```python
from build123d import *

# Parameters (mm, degrees)
SKETCH010_W     = 19.05
SKETCH010_H     = 25.4
PAD006_DEPTH    = 25.4
POCKET002_DEPTH = 25.401
SKETCH012_W     = 15.05
SKETCH012_H     = 23.4
POCKET003_DEPTH = 23.4
POCKET004_DEPTH = 19.051
FILLET003_R     = 1
FILLET004_R     = 0.5


with BuildPart() as part:
    # Sketch010 → Pad006 (new body)
    with BuildSketch(Plane.XY):
        Rectangle(SKETCH010_W, SKETCH010_H)
        with BuildLine():
            ThreePointArc((2.6035, 6.35), (0, 8.9535), (-2.6035, 6.35))
            Line((-2.6035, 6.35), (-2.6035, -6.35))
            ThreePointArc((-2.6035, -6.35), (0, -8.9535), (2.6035, -6.35))
            Line((2.6035, -6.35), (2.6035, 6.35))
        make_face(mode=Mode.SUBTRACT)
    extrude(amount=PAD006_DEPTH)

    # Sketch011 (on Face4 of Pad006) → Pocket002 (cut, through all)
    with BuildSketch(Plane.XZ.offset(12.7)):
        with BuildLine():
            ThreePointArc((2.6035, 19.05), (0, 21.6535), (-2.6035, 19.05))
            Line((-2.6035, 19.05), (-2.6035, 6.35))
            ThreePointArc((-2.6035, 6.35), (0, 3.7465), (2.6035, 6.35))
            Line((2.6035, 6.35), (2.6035, 19.05))
        make_face()
    extrude(amount=-POCKET002_DEPTH, mode=Mode.SUBTRACT)

    # Sketch012 (on Face5 of Pocket002) → Pocket003 (cut)
    with BuildSketch(Plane.XY.offset(25.4)):
        with Locations((0, -1)):
            Rectangle(SKETCH012_W, SKETCH012_H)
    extrude(amount=-POCKET003_DEPTH, mode=Mode.SUBTRACT)

    # Sketch013 (on Face9 of Pocket003) → Pocket004 (cut, through all)
    with BuildSketch(Plane(origin=(-9.525, 0, 0), x_dir=(0, -1, 0), z_dir=(-1, 0, 0))):
        Polygon((-10.7, 25.4), (12.7, 2), (12.7, 25.4), align=None)
    extrude(amount=-POCKET004_DEPTH, mode=Mode.SUBTRACT)

    # Fillet003
    fillet003_edges = [part.edges().sort_by_distance(p)[0] for p in [
        (0, -12.7, 0),
        (0, 12.7, 25.4),
        (9.525, -1, 13.7),
        (9.525, 12.7, 12.7),
        (9.525, 0, 0),
        (0, 12.7, 0),
        (-9.525, -1, 13.7),
        (9.525, -12.7, 1),
        (-9.525, -12.7, 1),
        (9.525, 11.7, 25.4),
        (-9.525, 11.7, 25.4),
        (-9.525, 0, 0),
        (-9.525, 12.7, 12.7),
    ]]
    fillet(fillet003_edges, radius=FILLET003_R)

    # Fillet004
    fillet004_edges = [part.edges().sort_by_distance(p)[0] for p in [
        (0, -12.7, 2),
        (0, 10.7, 25.4),
        (2.6035, 0, 2),
        (2.6035, 10.7, 12.7),
        (0, 12.7, 21.6535),
        (0, -8.9535, 0),
    ]]
    fillet(fillet004_edges, radius=FILLET004_R)


solid = part.part
```
Input: part model. Units: mm. Frame: model coordinates. A direction names the side the tool comes from. Give positions to 0.01 mm unless a question says otherwise; leave off trailing zeros. Order: outer loops, then holes, each group sorted by start corner. A loop starts at its lowest first (then second) coordinate and runs counter-clockwise, first axis right, second up. Notation, with made-up numbers: (84, 4) -> (103, 4) arc R23 ccw to (103, 22) -> close; hole circle Ø3 at (87, -6.5). An arc over 180 degrees is marked (long way). Write each question's results on one line, items separated by ' | '. Start each with the question number.
Item 1: Set-up query: faces 1 (the flat face through (4, 12.7, 13)), 2 (the flat face through (2.604, 0, 1)), 3 (the cylindrical face through (-0.057, 11.693, 3.747)), 4 (the flat face through (-7.525, 2, 11)). Return all of +Z, -Z, +X, -X, +Y, -Y with unobstructed straight access to the full face (end or side cutting, diameter ignored); none if empty.
Item 2: Line query: line 1 (X direction, y = 5.25, z = 12.75) (3 decimals); line 2 (Z direction, x = -7, y = -8.5); line 3 (Y direction, x = 2.5, z = 3). Output: solid intervals per line, ascending.
Item 3: Mould query, pull axis X, two halves, no side actions, for faces 5 (the cylindrical face through (0.119, 12.399, 0.285)), 6 (the cylindrical face through (-0.057, -8.953, 0.993)), 7 (the cylindrical face through (-9.24, -0.951, 13.324)). Classes: pulls with the +X half, pulls with the -X half, needs draft (parallel to the pull), parting line crosses it, or undercut.
Item 4: Cut plane A-A on x = 0. Return the cut outline in (y, z).
Item 5: Cut plane B-B on x = -4.25. Return the cut outline in (y, z).
Item 6: Contact query for flat-ended pins moving along their axis: P1, Ø4.5, axis at x = -1, z = 11, coming from the -Y side; P2, Ø2, axis at x = 3.5, y = 3.5, coming from the +Z side; P3, Ø6, axis at x = -7, y = -8.5, coming from the +Z side. Output: stop coordinate, or through.
Established:
1) face 1: +Z, -Z, +X, -X, +Y | face 2: +Z, -Z | face 3: +Y, -Y | face 4: +Z, -Y
2) line 1: -9.525 to -7.525, 7.525 to 9.525 | line 2: 0 to 2 | line 3: 10.7 to 12.7
3) face 5: needs draft | face 6: undercut | face 7: pulls with the -X half
4) outline: (-12.7, 1) arc R1 ccw to (-11.7, 0) -> (-9.45, 0) arc R0.5 ccw to (-8.95, 0.5) -> (-8.95, 1.5) arc R0.5 ccw to (-9.45, 2) -> (-12.2, 2) arc R0.5 ccw to (-12.7, 1.5) -> close; (8.95, 0.5) arc R0.5 ccw to (9.45, 0) -> (11.7, 0) arc R1 ccw to (12.7, 1) -> (12.7, 3.25) arc R0.5 ccw to (12.2, 3.75) -> (11.2, 3.75) arc R0.5 ccw to (10.7, 3.25) -> (10.7, 2) -> (9.45, 2) arc R0.5 ccw to (8.95, 1.5) -> close; (10.7, 22.15) arc R0.5 ccw to (11.2, 21.65) -> (12.2, 21.65) arc R0.5 ccw to (12.7, 22.15) -> (12.7, 24.4) arc R1 ccw to (11.7, 25.4) -> (11.2, 25.4) arc R0.5 ccw to (10.7, 24.9) -> close
5) outline: (-12.7, 1) arc R1 ccw to (-11.7, 0) -> (11.7, 0) arc R1 ccw to (12.7, 1) -> (12.7, 24.4) arc R1 ccw to (11.7, 25.4) -> (11.2, 25.4) arc R0.5 ccw to (10.7, 24.9) -> (10.7, 2) -> (-12.2, 2) arc R0.5 ccw to (-12.7, 1.5) -> close
6) P1: y = 10.7 | P2: z = 2 | P3: z = 9.15
